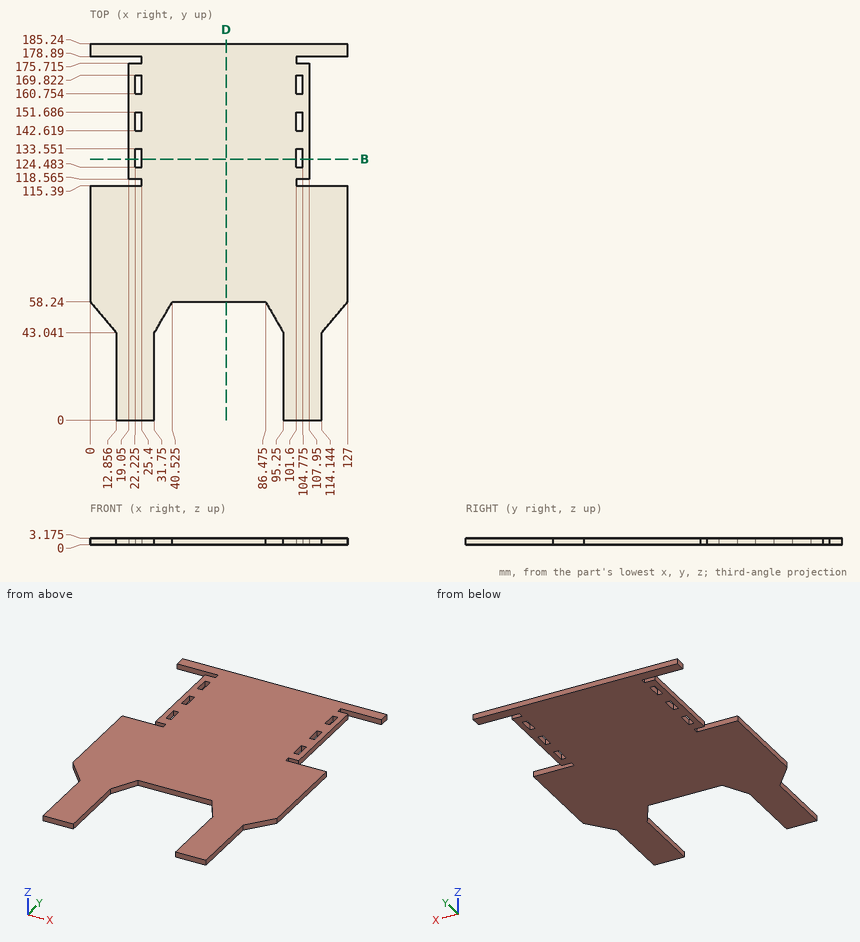
Answer from the drawing. Dimensions are ordinates in mm from the lowest x, y and z of the part. Coordinates: 2 decimals unless noted, no trailing zeros. Write each loop counter-clockwise with the first axis right and the second up, starting at its lowest first coordinate (ties: lowest second). Pieces come first, ordered by that corner, then holes. Notation, with made-up numbers: (-21.5, 83) -> (-4.5, 83) arc R35 ccw to (-4.5, 118) -> close; hole circle Ø10 at (16, 79). An arc over 180 degrees is marked (long way). One line per question, with ' | ' between items.
1. Straight lines are drawn through the part: line 1 (Y direction, x = 105, z = 2.7) (1 decimal); line 2 (X direction, y = 34.5, z = 2.65); line 3 (X direction, y = 170, z = 2.2). For each, find the intervals that lie inside material, in ascending order.
Verdict:
line 1: y = 0 to 115.4, 118.6 to 175.7, 178.9 to 185.2 | line 2: x = 12.86 to 31.75, 95.25 to 114.14 | line 3: x = 19.05 to 107.95
2. Section D-D (x = 67) is taken. Determine the outline of the cut face in (y, z) (1 decimal), and give its area (3 significant figures).
Verdict:
outline: (58.2, 0) -> (185.2, 0) -> (185.2, 3.2) -> (58.2, 3.2) -> close | area: 403 mm^2
3. Section B-B (y = 128.5) is taken. State how many separate pieces and enclosed holes the cut face has, and give its area (3 significant figures).
Verdict:
separate pieces: 3 | enclosed holes: 0 | area: 262 mm^2
4. Given pin 1 Ø1 at (x, z) = (23.5, 1.5) entering from -Y; pin 2 Ø1 at (y, z) = (14, 2) entering from +X; pin 3 Ø1 at (y, z) = (129, 2.5) entering from +X; pin 4 Ø1 at (y, z) = (148.5, 1) entering from -X, each flat-ended and moving along its own axis, determine where each tip first touches the part or whether it passes through.
Verdict:
pin 1: stops at y = 0 | pin 2: stops at x = 114.14 | pin 3: stops at x = 107.95 | pin 4: stops at x = 19.05
